CAD build for the part. Positions are in the model's coordinates, mm. A direction names the side the tool comes from. Coordinates: 2 decimals unless noted, no trailing zeros. Loops run counter-clockwise (first coordinate to the right, second up) from the corner with the lowest first, then second, coordinate; pieces in that order, holes last. Notation, with made-up numbers: (62, 39) -> (114, 39) arc R17 ccw to (114, 57) -> close; hole circle Ø1 at (78.5, 63.25). An arc over 180 degrees is marked (long way). Return JSON: item names as keys, results as strings. Group by question number.
(1) Saw through at A-A on x = 0. Write the cut outline in (y, z).
(2) Probe L1, parallel to X at y = 16.25, z = 13.81; L2, parallel to Y at x = -1, z = 13; L3, parallel to Z at x = -4.75, y = 5. List the from-to ranges inside material, lowest first.
(3) Saw through at D-D on y = 5.5. Write the cut outline in (x, z).
(4) Saw through at B-B on z = -13.81. Write the cut outline in (x, y), then the cut area to 3 significant figures.
(5) Flat gauge pins, fed straight in: pin 1 Ø2 at (x, y) = (0, 19.5) entering from -Z; pin 2 Ø1 at (x, z) = (4.5, 12.5) entering from -Y; pin 3 Ø4 at (x, z) = (1.5, 14.5) entering from +Y; pin 4 Ø3 at (x, z) = (2, 4.5) entering from +Y. Where does each tip first touch, or does it go through?
(6) Tool access for faces 4 (the face through (0, 15.7, 15)), 5 (the face through (0, 22.5, -7)), 6 (the face through (0, 22, 11.55)): list every direction of +Z, -Z, +X, -X, +Y, -Y with a clear straight run to the whole face (end or side of a thin tool).
(7) Mould opens along X. For faces 1 (the face through (-0.61, 16.97, -14.6)), 2 (the face through (-0.084, 28.526, 7.224)), 3 (the face through (0, 8, -11.55)) say: pulls with the +X half, pulls with the -X half, needs draft (parallel to the pull), parting line crosses it, or undercut.
(8) Saw through at C-C on x = 2.75. Write the cut outline in (y, z), then the cut area to 3 significant figures.
```python
from build123d import *

# Parameters (mm, degrees)
SKETCH2_W           = 12.6
SKETCH2_H           = 23.1
BOSS_EXTRUDE1_DEPTH = 15.7
SKETCH3_W           = 12.6
SKETCH3_H           = 32.5
BOSS_EXTRUDE2_DEPTH = 2.5
SKETCH4_W           = 12.6
SKETCH4_H           = 23.1
BOSS_EXTRUDE3_DEPTH = 4.3
SKETCH5_W           = 12.6
SKETCH5_H           = 13
BOSS_EXTRUDE4_DEPTH = 4.3
SKETCH7_R           = 1.912877934
BOSS_EXTRUDE6_DEPTH = 3.5
SKETCH8_R           = 1
CUT_EXTRUDE1_DEPTH  = 3.5


with BuildPart() as part:
    # Sketch2 → Boss-Extrude1 (new body)
    with BuildSketch(Plane(origin=(0, 0, 0), x_dir=(1, 0, 0), z_dir=(0, 1, 0))):
        Rectangle(SKETCH2_W, SKETCH2_H)
    extrude(amount=BOSS_EXTRUDE1_DEPTH)

    # Sketch3 → Boss-Extrude2 (add)
    with BuildSketch(Plane(origin=(0, 15.7, 0), x_dir=(1, 0, 0), z_dir=(0, 1, 0))):
        Rectangle(SKETCH3_W, SKETCH3_H)
    extrude(amount=BOSS_EXTRUDE2_DEPTH)

    # Sketch4 → Boss-Extrude3 (add)
    with BuildSketch(Plane(origin=(0, 18.2, 0), x_dir=(1, 0, 0), z_dir=(0, 1, 0))):
        Rectangle(SKETCH4_W, SKETCH4_H)
    extrude(amount=BOSS_EXTRUDE3_DEPTH)

    # Sketch5 → Boss-Extrude4 (add)
    with BuildSketch(Plane(origin=(0, 22.5, 0), x_dir=(1, 0, 0), z_dir=(0, 1, 0))):
        with Locations((0, -5.05)):
            Rectangle(SKETCH5_W, SKETCH5_H)
    extrude(amount=BOSS_EXTRUDE4_DEPTH)

    # Sketch7 → Boss-Extrude6 (add)
    with BuildSketch(Plane(origin=(0, 26.8, 0), x_dir=(1, 0, 0), z_dir=(0, 1, 0))):
        with Locations(Location((0, -5.312938635, 0), (0, 0, 90))):
            Circle(SKETCH7_R)
    extrude(amount=BOSS_EXTRUDE6_DEPTH)

    # Sketch8 → Cut-Extrude1 (cut)
    with BuildSketch(Plane(origin=(0, 18.2, 0), x_dir=(1, 0, 0), z_dir=(0, 1, 0))):
        with Locations(Location((0, 13.81, 0), (0, 0, 270))):
            Circle(SKETCH8_R)
        with Locations(Location((0, -13.81, 0), (0, 0, 270))):
            Circle(SKETCH8_R)
    extrude(amount=-CUT_EXTRUDE1_DEPTH, mode=Mode.SUBTRACT)


solid = part.part
```
Geometry results:
{
 "1": {"outline": "(0, -11.55) -> (15.7, -11.55) -> (15.7, -12.81) -> (18.2, -12.81) -> (18.2, -11.55) -> (22.5, -11.55) -> (22.5, -1.45) -> (26.8, -1.45) -> (26.8, 3.4) -> (30.3, 3.4) -> (30.3, 7.23) -> (26.8, 7.23) -> (26.8, 11.55) -> (18.2, 11.55) -> (18.2, 12.81) -> (15.7, 12.81) -> (15.7, 11.55) -> (0, 11.55) -> close; (15.7, -16.25) -> (18.2, -16.25) -> (18.2, -14.81) -> (15.7, -14.81) -> close; (15.7, 14.81) -> (18.2, 14.81) -> (18.2, 16.25) -> (15.7, 16.25) -> close"},
 "2": {"L1": "-6.3 to -1, 1 to 6.3", "L2": "15.7 to 18.2", "L3": "-11.55 to 11.55"},
 "3": {"outline": "(-6.3, -11.55) -> (6.3, -11.55) -> (6.3, 11.55) -> (-6.3, 11.55) -> close"},
 "4": {"outline": "(-6.3, 15.7) -> (-1, 15.7) -> (-1, 18.2) -> (-6.3, 18.2) -> close; (1, 15.7) -> (6.3, 15.7) -> (6.3, 18.2) -> (1, 18.2) -> close", "area": "26.5 mm²"},
 "5": {"pin 1": "z = -11.55", "pin 2": "y = 15.7", "pin 3": "y = 18.2", "pin 4": "y = 30.3"},
 "6": {"face 4": "+Z, +X, -X, -Y", "face 5": "-Z, +X, -X, +Y", "face 6": "+Z, +X, -X, +Y"},
 "7": {"face 1": "undercut", "face 2": "parting line crosses it", "face 3": "needs draft"},
 "8": {"outline": "(0, -11.55) -> (15.7, -11.55) -> (15.7, -16.25) -> (18.2, -16.25) -> (18.2, -11.55) -> (22.5, -11.55) -> (22.5, -1.45) -> (26.8, -1.45) -> (26.8, 11.55) -> (18.2, 11.55) -> (18.2, 16.25) -> (15.7, 16.25) -> (15.7, 11.55) -> (0, 11.55) -> close", "area": "599 mm²"}
}
